from build123d import *

# Parameters (mm, degrees)
SCHIZZO1_R                   = 1.5
ESTRUSIONE_ESTRUSIONE1_DEPTH = 1.35
RACCORDO2_R                  = 3
RACCORDO3_R                  = 3
RACCORDO4_R                  = 0.7


with BuildPart() as part:
    # Schizzo1 → Estrusione-Estrusione1 (new body)
    with BuildSketch(Plane(origin=(0, 0, 0), x_dir=(0, 0, -1), z_dir=(1, 0, 0))):
        with BuildLine():
            add(Edge.make_bspline(
                [(-7.501010101, -10.3), (-10.845030199, -9.13986581), (-13.865102381, -7.304364218), (-17.601010101, -6.594005849)],
                knots=[0.271280726, 0.271280726, 0.271280726, 0.271280726, 0.852483684, 0.852483684, 0.852483684, 0.852483684], degree=3))
            add(Edge.make_bspline(
                [(-2.501010101, -11.3), (-4.308742426, -11.235865063), (-5.940164296, -10.841501107), (-7.501010101, -10.3)],
                knots=[0, 0, 0, 0, 0.271280726, 0.271280726, 0.271280726, 0.271280726], degree=3))
            Line((-2.501010101, -11.3), (1.498989899, -11.3))
            ThreePointArc((1.498989899, -11.3), (11.398989899, 0), (1.498989899, 11.3))
            Line((1.498989899, 11.3), (-2.501010101, 11.3))
            add(Edge.make_bspline(
                [(-2.501010101, 11.3), (-4.209338931, 11.338090952), (-5.850739142, 10.914740779), (-7.501010101, 10.3)],
                knots=[0, 0, 0, 0, 0.293888871, 0.293888871, 0.293888871, 0.293888871], degree=3))
            add(Edge.make_bspline(
                [(-7.501010101, 10.3), (-10.658273676, 9.123890914), (-13.848006436, 7.247243694), (-17.601010101, 6.561146452)],
                knots=[0.293888871, 0.293888871, 0.293888871, 0.293888871, 0.856150858, 0.856150858, 0.856150858, 0.856150858], degree=3))
            Line((-17.601010101, 6.561146452), (-17.601010101, 0))
            Line((-17.601010101, 0), (-17.601010101, -6.594005849))
        make_face()
        with Locations(Location((5, -6, 0), (0, 0, 180))):
            Circle(SCHIZZO1_R, mode=Mode.SUBTRACT)
        with BuildLine():
            ThreePointArc((-10.5, 0), (-12, -1.5), (-13.5, 0))
            ThreePointArc((-13.5, 0), (-12, 1.5), (-10.5, 0))
        make_face(mode=Mode.SUBTRACT)
        Polygon((-7.9, -2.9), (-7.9, 0), (-7.9, 2.9), (-1.901010101, 2.9), (-1.901010101, 3.4), (2.098989899, 3.4), (2.098989899, 2.9), (7.898989899, 2.9), (7.898989899, -2.9), (2.098989899, -2.9), (2.098989899, -3.4), (-1.901010101, -3.4), (-1.901010101, -2.9), align=None, mode=Mode.SUBTRACT)
        with Locations(Location((5, 6, 0), (0, 0, 180))):
            Circle(SCHIZZO1_R, mode=Mode.SUBTRACT)
    extrude(amount=ESTRUSIONE_ESTRUSIONE1_DEPTH)

    # Raccordo2
    raccordo2_edges = [part.edges().sort_by_distance(p)[0] for p in [
        (0.675, -6.594005849, 17.601010101),
    ]]
    fillet(raccordo2_edges, radius=RACCORDO2_R)

    # Raccordo3
    raccordo3_edges = [part.edges().sort_by_distance(p)[0] for p in [
        (0.675, 6.561146452, 17.601010101),
    ]]
    fillet(raccordo3_edges, radius=RACCORDO3_R)

    # Raccordo4
    raccordo4_edges = [part.edges().sort_by_distance(p)[0] for p in [
        (0.675, -2.9, -7.898989899),
        (0.675, 2.9, -7.898989899),
        (0.675, 2.9, 7.9),
        (0.675, -2.9, 7.9),
    ]]
    fillet(raccordo4_edges, radius=RACCORDO4_R)


solid = part.part
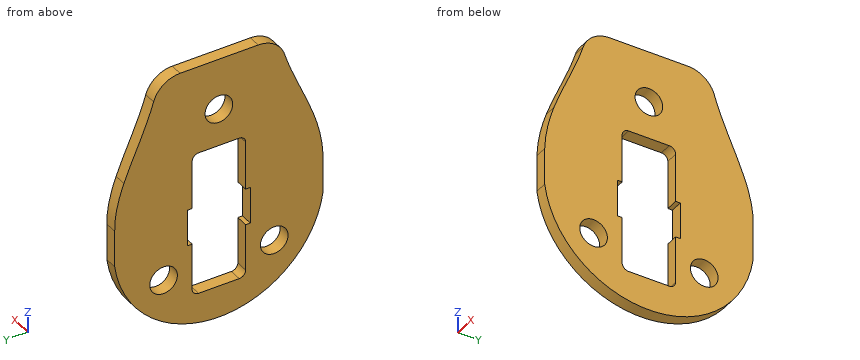
Input: part model. Units: mm. Frame: model coordinates. Give positions to 0.01 mm unless a question says otherwise; leave off trailing zeros. Write each loop counter-clockwise with the first axis right and the second up, starting at its lowest first coordinate (ties: lowest second). Pieces come first, ordered by that corner, then holes. Notation, with made-up numbers: M 47.5,61.25 L 85.5,61.25 A18 cw 85.5,79.25 Z; hole C 32.25,-18 d2. An arc over 180 degrees is marked long. Write item = value, one per line. Start each with the question number.
1) Cut plane D-D on z = -8.75. Return the cut outline in (x, y).
2) First-contact query: pin 1 Ø0.7 at (x, z) = (0.5, -4.5) entering from +Y. Flat tip, straight axial feed; report the tip coordinate or a pass-through.
3) Cut plane C-C on x = 0.7. Count the separate pieces of the cut face and the enclosed holes in it, then the cut area to 3 significant figures.
4) Cut plane A-A on y = 0. Return the cut outline in (x, z), then the cut area to 3 significant figures.
5) Cut plane B-B on z = -5. Return the cut outline in (x, y).
6) Material intervals for line 1 along Y through (x, z) = (0.65, 2.25); line 2 along Y through (x, z) = (0.25, 0); line 3 along Y through (x, z) = (0.5, -5), sorted ascending. Write a range as [from, to].
Solved:
q1.outline = M 0,-7.31 L 1.35,-7.31 L 1.35,7.31 L 0,7.31 Z
q2.pin_1 = 10.62
q3.separate_pieces = 1
q3.enclosed_holes = 4
q3.area = 419 mm2
q4.outline = M 0,-11.4 L 1.35,-11.4 L 1.35,-7.9 L 0,-7.9 Z; M 0,7.9 L 1.35,7.9 L 1.35,10.5 L 0,10.5 Z; M 0,13.5 L 1.35,13.5 L 1.35,17.6 L 0,17.6 Z
q4.area = 13.8 mm2
q5.outline = M 0,-10.24 L 1.35,-10.24 L 1.35,-7.5 L 0,-7.5 Z; M 0,-4.5 L 1.35,-4.5 L 1.35,-2.9 L 0,-2.9 Z; M 0,2.9 L 1.35,2.9 L 1.35,4.5 L 0,4.5 Z; M 0,7.5 L 1.35,7.5 L 1.35,10.24 L 0,10.24 Z
q6.line_1 = [-11.3, -2.9], [2.9, 11.3]
q6.line_2 = [-11.3, -3.4], [3.4, 11.3]
q6.line_3 = [-10.24, -7.5], [-4.5, -2.9], [2.9, 4.5], [7.5, 10.24]
